Autodesk Inventor part; units mm, degrees
ref_plane "to_bm_terminals_XY" through (0, -8.9154, 0) normal (0, -1, 0) x (1, 0, 0)
ref_plane "to_bm_terminals_YZ" through (0, -8.9154, 0) normal (1, 0, 0) x (0, 0, 1)
ref_plane "to_bm_terminals_ZX" through (0, -8.9154, 0) normal (0, 0, 1) x (0, -1, 0)
sketch "Sketch_1" plane through (0, 0, 0) normal (0, 1, 0) x (-1, 0, 0)
  line L0 (3.9497, 5.1435) -> (3.9497, 6.3754)
  arc A0 (3.9497, 6.3754) -> (3.8227, 6.5024) centre (3.8227, 6.3754) ccw
  line L1 (3.8227, 6.5024) -> (-3.8227, 6.5024)
  arc A1 (-3.8227, 6.5024) -> (-3.9497, 6.3754) centre (-3.8227, 6.3754) ccw
  line L2 (-3.9497, 6.3754) -> (-3.9497, 5.1435)
  line L3 (-3.9497, 5.1435) -> (-3.6957, 5.1435)
  line L4 (-3.6957, 5.1435) -> (-3.6957, 2.9397)
  line L5 (-3.6957, 2.9397) -> (-2.6797, 2.7606)
  line L6 (-2.6797, 2.7606) -> (-2.6797, 1.9384)
  line L7 (-2.6797, 1.9384) -> (-3.6957, 1.7593)
  line L8 (-3.6957, 1.7593) -> (-3.6957, -1.7593)
  line L9 (-3.6957, -1.7593) -> (-2.6797, -1.9384)
  line L10 (-2.6797, -1.9384) -> (-2.6797, -2.7606)
  line L11 (-2.6797, -2.7606) -> (-3.6957, -2.9397)
  line L12 (-3.6957, -2.9397) -> (-3.6957, -5.1435)
  line L13 (-3.6957, -5.1435) -> (-3.9497, -5.1435)
  line L14 (-3.9497, -5.1435) -> (-3.9497, -6.3754)
  arc A2 (-3.9497, -6.3754) -> (-3.8227, -6.5024) centre (-3.8227, -6.3754) ccw
  line L15 (-3.8227, -6.5024) -> (3.8227, -6.5024)
  arc A3 (3.8227, -6.5024) -> (3.9497, -6.3754) centre (3.8227, -6.3754) ccw
  line L16 (3.9497, -6.3754) -> (3.9497, -5.1435)
  line L17 (3.9497, -5.1435) -> (3.6957, -5.1435)
  line L18 (3.6957, -5.1435) -> (3.6957, -2.9397)
  line L19 (3.6957, -2.9397) -> (2.6797, -2.7606)
  line L20 (2.6797, -2.7606) -> (2.6797, -1.9384)
  line L21 (2.6797, -1.9384) -> (3.6957, -1.7593)
  line L22 (3.6957, -1.7593) -> (3.6957, 1.7593)
  line L23 (3.6957, 1.7593) -> (2.6797, 1.9384)
  line L24 (2.6797, 1.9384) -> (2.6797, 2.7606)
  line L25 (2.6797, 2.7606) -> (3.6957, 2.9397)
  line L26 (3.6957, 2.9397) -> (3.6957, 5.1435)
  line L27 (3.6957, 5.1435) -> (3.9497, 5.1435)
extrude "Extrusion1" add sketch "Sketch_1" against normal blind 9.1694
sketch "Sketch_2" plane through (0, 0, 0) normal (0, 1, 0) x (-1, 0, 0)
  line L0 (3.6957, 6.2484) -> (-3.6957, 6.2484)
  line L1 (-3.6957, 6.2484) -> (-3.6957, -6.2484)
  line L2 (-3.6957, -6.2484) -> (3.6957, -6.2484)
  line L3 (3.6957, -6.2484) -> (3.6957, 6.2484)
extrude "Extrusion2" add sketch "Sketch_2" along normal blind 3.5814
sketch "Sketch_28" plane through (0, 0, 0) normal (0, 1, 0) x (-1, 0, 0)
  line L0 (3.6957, 6.2484) -> (-3.6957, 6.2484)
  line L1 (-3.6957, 6.2484) -> (-3.6957, -6.2484)
  line L2 (-3.6957, -6.2484) -> (3.6957, -6.2484)
  line L3 (3.6957, -6.2484) -> (3.6957, 6.2484)
extrude "Extrusion3" add sketch "Sketch_28" against normal blind 6.7564
sketch "Sketch_9" plane through (0, -9.1694, 0) normal (0, 1, 0) x (1, 0, 0)
  arc A0 (-2.286, 2.3194) -> (-2.032, 2.0654) centre (-2.032, 2.3194) ccw
  line L0 (-2.032, 2.0654) -> (2.032, 2.0654)
  arc A1 (2.032, 2.0654) -> (2.286, 2.3194) centre (2.032, 2.3194) ccw
  line L1 (2.286, 2.3194) -> (2.286, 2.3796)
  arc A2 (2.286, 2.3796) -> (2.032, 2.6336) centre (2.032, 2.3796) ccw
  line L2 (2.032, 2.6336) -> (-2.032, 2.6336)
  arc A3 (-2.032, 2.6336) -> (-2.286, 2.3796) centre (-2.032, 2.3796) ccw
  line L3 (-2.286, 2.3796) -> (-2.286, 2.3194)
extrude "Extrusion4" add sketch "Sketch_9" against normal blind 0.508
sketch "Sketch_10" plane through (0, -9.1694, 0) normal (0, 1, 0) x (1, 0, 0)
  line L0 (-2.286, -2.3194) -> (-2.286, -2.3796)
  arc A0 (-2.286, -2.3796) -> (-2.032, -2.6336) centre (-2.032, -2.3796) ccw
  line L1 (-2.032, -2.6336) -> (2.032, -2.6336)
  arc A1 (2.032, -2.6336) -> (2.286, -2.3796) centre (2.032, -2.3796) ccw
  line L2 (2.286, -2.3796) -> (2.286, -2.3194)
  arc A2 (2.286, -2.3194) -> (2.032, -2.0654) centre (2.032, -2.3194) ccw
  line L3 (2.032, -2.0654) -> (-2.032, -2.0654)
  arc A3 (-2.032, -2.0654) -> (-2.286, -2.3194) centre (-2.032, -2.3194) ccw
extrude "Extrusion5" add sketch "Sketch_10" against normal blind 0.508
ref_plane "to_bm_terminals_XY" through (0, -8.9154, 0) normal (0, -1, 0) x (1, 0, 0)
ref_plane "to_bm_terminals_YZ" through (0, -8.9154, 0) normal (1, 0, 0) x (0, 0, 1)
ref_plane "to_bm_terminals_ZX" through (0, -8.9154, 0) normal (0, 0, 1) x (0, -1, 0)
ref_plane "to_bodycover_XY" through (0, 3.5814, 0) normal (0, -1, 0) x (1, 0, 0)
ref_plane "to_bodycover_YZ" through (0, 3.5814, 0) normal (1, 0, 0) x (0, 0, 1)
ref_plane "to_bodycover_ZX" through (0, 3.5814, 0) normal (0, 0, 1) x (0, -1, 0)
ref_plane "to_dummy_XY" through (0, 0, 0) normal (0, -1, 0) x (1, 0, 0)
ref_plane "to_dummy_YZ" through (0, 0, 0) normal (1, 0, 0) x (0, 0, 1)
ref_plane "to_dummy_ZX" through (0, 0, 0) normal (0, 0, 1) x (0, -1, 0)
properties part number "MB2011-body"
Input: part model. Units: mm. Frame: model coordinates. A direction names the side the tool comes from. Round coordinates to 2 decimals unless told otherwise and drop trailing zeros. Order: outer loops, then holes, each group sorted by start corner. A loop starts at its lowest first (then second) coordinate and runs counter-clockwise, first axis right, second up. Notation, with made-up numbers: (10.5, -31.75) - (69.5, -31.75) arc R24 cw to (69.5, -7.75) - close; hole circle Ø11 at (23.25, -17). An arc over 180 degrees is marked (long way). Use a Markdown table: item, result.
1. First-contact query: pin 1 (1.5 mm diameter, centred on y = 1.5, z = -1.5, fed in from -X); pin 2 (2 mm diameter, centred on x = 0.5, z = 1, fed in from -Y); pin 3 (0.6 mm diameter, centred on x = 0, y = -9.5, fed in from -Z). Flat tips, straight axial feed; report the tip coordinate or a pass-through.
Evaluation:
| item | result |
|---|---|
| pin 1 | x = -3.7 |
| pin 2 | y = -9.17 |
| pin 3 | z = -2.63 |
2. Mould query, pull axis Z, two halves, no side actions, for faces 1 (the face through (-3.19, -7.95, 1.85)), 2 (the face through (0, 3.581, 0)), 3 (the face through (0, 2, -6.248)). Classes: +Z half, -Z half, draft (parallel to the pull), parting line (faces both ways), or undercut.
Evaluation:
| item | result |
|---|---|
| face 1 | undercut |
| face 2 | draft |
| face 3 | -Z half |
3. Section C-C on z = 0.25. Return the cut outline in (x, y).
Evaluation:
| item | result |
|---|---|
| outline | (-3.7, -9.17) - (3.7, -9.17) - (3.7, 3.58) - (-3.7, 3.58) - close |
4. Material intervals for probe 1 along X at (y, z) = (1.5, 1.75); probe 2 along Z at (x, y) = (1, 1); probe 3 along Y at (x, z) = (-0.25, -2), sorted ascending.
Evaluation:
| item | result |
|---|---|
| probe 1 | -3.7 to 3.7 |
| probe 2 | -6.25 to 6.25 |
| probe 3 | -9.17 to 3.58 |
5. Section B-B on x = -1.25. Return the cut outline in (y, z), then the cut area to 3 significant figures.
Evaluation:
| item | result |
|---|---|
| outline | (-9.68, -2.63) - (-9.17, -2.63) - (-9.17, -6.5) - (0, -6.5) - (0, -6.25) - (3.58, -6.25) - (3.58, 6.25) - (0, 6.25) - (0, 6.5) - (-9.17, 6.5) - (-9.17, 2.63) - (-9.68, 2.63) - (-9.68, 2.07) - (-9.17, 2.07) - (-9.17, -2.07) - (-9.68, -2.07) - close |
| area | 165 mm^2 |
6. Access query for faces 4 (the face through (0, 2, 6.248)), 5 (the face through (3.18, -7.95, -2.85)), 6 (the face through (-3.2, -6.756, -2.3)). Directions: +Z, -Z, +X, -X, +Y, -Y. A direction counts if a zero-diameter tool reaches every point of the face in a straight line with its end or side. Return the directions, or none.
Evaluation:
| item | result |
|---|---|
| face 4 | +Z, +X, -X, +Y |
| face 5 | +X, -Y |
| face 6 | -X, -Y |
7. Section D-D on y = -3.75. Return the cut outline in (x, z), then the cut area to 3 significant figures.
Evaluation:
| item | result |
|---|---|
| outline | (-3.95, -6.38) arc R0.13 ccw to (-3.82, -6.5) - (3.82, -6.5) arc R0.13 ccw to (3.95, -6.38) - (3.95, -5.14) - (3.7, -5.14) - (3.7, 5.14) - (3.95, 5.14) - (3.95, 6.38) arc R0.13 ccw to (3.82, 6.5) - (-3.82, 6.5) arc R0.13 ccw to (-3.95, 6.38) - (-3.95, 5.14) - (-3.7, 5.14) - (-3.7, -5.14) - (-3.95, -5.14) - close |
| area | 97.5 mm^2 |
